Model file for the job. Use its own axes, mm. A direction names the side the tool comes from. Round coordinates to 2 decimals unless told otherwise and drop trailing zeros. Order: outer loops, then holes, each group sorted by start corner. A loop starts at its lowest first (then second) coordinate and runs counter-clockwise, first axis right, second up. Notation, with made-up numbers: (-26.5, 10.5) - (4.5, 10.5) arc R31 cw to (4.5, 49.5) - close; hole circle Ø11 at (24.25, -34.5). An arc over 180 degrees is marked (long way). Put each result on its own line as item: value. Start each with the question number.
Item 1: Saw through at A-A on x = 53. List the corners of the cut face in (y, z).
Item 2: Which spindle directions (+Z, -Z, +X, -X, +Y, -Y) get a long thin tool onto all of the face, cutting with end or side? Do faces 5 (the face through (-37, -14.246, -31)), 6 (the face through (18, -24, 39.1)), 7 (the face through (55, -29.764, 16)). Say none if no direction does.
Item 3: Probe probe 1 along Z at (x, y) = (19.5, -9.5); probe 2 along Z at (x, y) = (33, -22.5); probe 3 along X at (y, z) = (-20, -27.5). List the from-to ranges inside material, lowest first.
Item 4: Saw through at D-D on y = -25. List the corners of the cut face in (x, z).
Item 5: Saw through at C-C on z = 16.5. List the corners of the cut face in (x, y).
Item 6: Pin check, flat tips, straight feed: pin 1 Ø1.5 at (x, y) = (13.5, -27) entering from +Z; pin 2 Ø10 at (x, y) = (-44, -28) entering from -Z; pin 3 Ø3.5 at (y, z) = (-35, -34) entering from -X. Stop position of each tip, or through.
Item 7: Mould opens along Z. For faces 1 (the face through (55, -22.764, 16)), 2 (the face through (-1, -50.8, 0)), 3 (the face through (55, -26, 9.693)), 4 (the face through (0.89, -1.43, -36.6)) say: pulls with the +Z half, pulls with the -Z half, needs draft (parallel to the pull), parting line crosses it, or undercut.
Item 8: Saw through at B-B on x = -4. List the corners of the cut face in (y, z), plus the area to 3 significant figures.
```python
from build123d import *

# Parameters (mm, degrees)
F0_W      = 127
F0_H      = 76.2
F1_DEPTH  = 50.8
F2_R      = 5
F3_R      = 5
F4_R      = 5
F5_W      = 7
F5_H      = 13.8
F6_DEPTH  = 16.4
F7_W      = 5.596507
F7_H      = 1.424566
F8_DEPTH  = 13.4
F9_W      = 45
F9_H      = 12
F10_DEPTH = 1
F11_R     = 3.85898
F12_DEPTH = 2
F13_W     = 53.570701
F13_H     = 22.736654
F14_DEPTH = 15
F15_W     = 33.673272
F15_H     = 8.921977
F16_DEPTH = 15


with BuildPart() as f1:
    # F0 (on Front) → F1 (new body)
    with BuildSketch(Plane.XZ):
        Rectangle(F0_W, F0_H)
    extrude(amount=F1_DEPTH)

    # F2
    f2_edges = [f1.edges().sort_by_distance(p)[0] for p in [
        (0, -50.8, 38.1),
    ]]
    fillet(f2_edges, radius=F2_R)

    # F3
    f3_edges = [f1.edges().sort_by_distance(p)[0] for p in [
        (0, 0, 38.1),
    ]]
    fillet(f3_edges, radius=F3_R)

    # F4
    f4_edges = [f1.edges().sort_by_distance(p)[0] for p in [
        (0, -50.8, -38.1),
        (0, 0, -38.1),
    ]]
    fillet(f4_edges, radius=F4_R)

    # F5 (on face) → F6 (cut)
    with BuildSketch(Plane.YZ.offset(63.5)):
        with Locations((-26.263526, 16.592734)):
            Rectangle(F5_W, F5_H)
    extrude(amount=-F6_DEPTH, mode=Mode.SUBTRACT)

    # F7 (on face) → F8 (cut)
    with BuildSketch(Plane.YZ.offset(63.5)):
        with Locations((-26.507245, 25.401587)):
            Rectangle(F7_W, F7_H)
    extrude(amount=-F8_DEPTH, mode=Mode.SUBTRACT)

    # F9 (on face) → F10 (cut)
    with BuildSketch(Plane.XY.offset(38.1)):
        with Locations((34.471648, -23.887878)):
            Rectangle(F9_W, F9_H)
    extrude(amount=-F10_DEPTH, mode=Mode.SUBTRACT)

    # F11 (on face) → F12 (join)
    with BuildSketch(Plane.XY.offset(37.1)):
        with Locations((17.887004, -23.616357)):
            Circle(F11_R)
    extrude(amount=F12_DEPTH)

    # F13 (on face) → F14 (cut)
    with BuildSketch(Plane(origin=(0, 0, -38.1), x_dir=(1, 0, 0), z_dir=(0, 0, -1))):
        with Locations((-36.71465, 25.614712)):
            Rectangle(F13_W, F13_H)
    extrude(amount=-F14_DEPTH, mode=Mode.SUBTRACT)

    # F15 (on face) → F16 (join)
    with BuildSketch(Plane(origin=(0, 0, -23.1), x_dir=(1, 0, 0), z_dir=(0, 0, -1))):
        with Locations((-26.765935, 25.326905)):
            Rectangle(F15_W, F15_H)
    extrude(amount=F16_DEPTH)


solid = f1.part
```
Results found:
1. outline: (-50.8, -33.1) arc R5 ccw to (-45.8, -38.1) - (-5, -38.1) arc R5 ccw to (0, -33.1) - (0, 33.1) arc R5 ccw to (-5, 38.1) - (-17.89, 38.1) - (-17.89, 37.1) - (-29.89, 37.1) - (-29.89, 38.1) - (-45.8, 38.1) arc R5 ccw to (-50.8, 33.1) - close; hole (-29.76, 9.69) - (-22.76, 9.69) - (-22.76, 23.49) - (-29.76, 23.49) - close; hole (-29.31, 24.69) - (-23.71, 24.69) - (-23.71, 26.11) - (-29.31, 26.11) - close
2. face 5: -Z, -X
2. face 6: +Z, +X, -X, +Y, -Y
2. face 7: +X
3. probe 1: z = -38.1 to 38.1
3. probe 2: z = -38.1 to 37.1
3. probe 3: x = -9.93 to 63.5
4. outline: (-63.5, -23.1) - (-43.6, -23.1) - (-43.6, -38.1) - (63.5, -38.1) - (63.5, 9.69) - (47.1, 9.69) - (47.1, 23.49) - (63.5, 23.49) - (63.5, 24.69) - (50.1, 24.69) - (50.1, 26.11) - (63.5, 26.11) - (63.5, 38.1) - (56.97, 38.1) - (56.97, 37.1) - (21.49, 37.1) - (21.49, 39.1) - (14.28, 39.1) - (14.28, 37.1) - (11.97, 37.1) - (11.97, 38.1) - (-63.5, 38.1) - close
5. outline: (-63.5, -50.8) - (63.5, -50.8) - (63.5, -29.76) - (47.1, -29.76) - (47.1, -22.76) - (63.5, -22.76) - (63.5, 0) - (-63.5, 0) - close
6. pin 1: stops at z = 37.1
6. pin 2: stops at z = -38.1
6. pin 3: stops at x = -9.93
7. face 1: undercut
7. face 2: needs draft
7. face 3: undercut
7. face 4: pulls with the -Z half
8. outline: (-50.8, -33.1) arc R5 ccw to (-45.8, -38.1) - (-5, -38.1) arc R5 ccw to (0, -33.1) - (0, 33.1) arc R5 ccw to (-5, 38.1) - (-45.8, 38.1) arc R5 ccw to (-50.8, 33.1) - close
8. area: 3,850 mm²
